The listing builds one solid part. Answer for the finished solid, in the listing's coordinates (mm). A direction names the side the tool comes from. Coordinates: 2 decimals unless noted, no trailing zeros. Loops run counter-clockwise (first coordinate to the right, second up) from the corner with the lowest first, then second, coordinate; pieces in that order, holes last. Notation, with made-up numbers: (-6, -3.5) - (41, -3.5) arc R17 ccw to (41, 3.5) - close; hole circle Ø8 at (5.25, 74). An arc over 180 degrees is marked (long way). Write each question's results on one line, items separated by ' | '. Start each with the question number.
(1) Consider line 1 (Z direction, x = 90, y = 10.5); line 2 (Y direction, x = 75, z = -9.5) (3 decimals); line 3 (X direction, y = 13.75, z = -15.5). Determine where each line is inside the solid, lowest interval first. Write a range as from..to.
(2) For faces 1 (the flat face through (0, 6, -15)), 2 (the flat face through (49, 0, -15)), 3 (the cylindrical face through (66, 12.54, -23.57)), 4 (the flat face through (14, 10, -15)), 5 (the cylindrical face through (72.5, 12.54, -15.16)), determine the directions among +Z, -Z, +X, -X, +Y, -Y from which every point of the face is accessible in a straight line to the end or side of a thin tool.
(3) Find section A-A on y = 12.75. Determine the outline of the cut face in (x, z).
(4) Find section C-C on x = 16. Determine the outline of the cut face in (y, z), then the cut area to 3 significant figures.
(5) Given pin 1 Ø2.5 at (y, z) = (12.5, -13.5) entering from +X, flat-ended and moving along its own axis, determine where the tip first touches the part or whether it passes through.
(6) Determine the mould class of faces 6 (the flat face through (50, 10, -15)), 7 (the flat face through (10, 13, -22.5)), 8 (the flat face through (100, 6, -15)) for opening direction X: released by +X, released by -X, zero draft, split by the parting line, or undercut.
(7) Find section B-B on z = -15. Determine the outline of the cut face in (x, y) (3 decimals).
(8) Find section D-D on x = 39. Determine the outline of the cut face in (y, z).
from build123d import *

# Parameters (mm, degrees)
SKETCH1_W           = 100
SKETCH1_H           = 30
BOSS_EXTRUDE1_DEPTH = 15
CUT_EXTRUDE1_DEPTH  = 5
SKETCH3_R           = 0.625
CUT_EXTRUDE2_DEPTH  = 30
CUT_EXTRUDE3_DEPTH  = 5


with BuildPart() as part:
    # Sketch1 → Boss-Extrude1 (new body)
    with BuildSketch(Plane(origin=(0, 0, 0), x_dir=(1, 0, 0), z_dir=(0, 1, 0))):
        with Locations((50, 15)):
            Rectangle(SKETCH1_W, SKETCH1_H)
    extrude(amount=BOSS_EXTRUDE1_DEPTH)

    # Sketch2 → Cut-Extrude1 (cut)
    with BuildSketch(Plane(origin=(0, 15, 0), x_dir=(1, 0, 0), z_dir=(0, 1, 0))):
        with BuildLine():
            Line((-20, 22.5), (20, 22.5))
            ThreePointArc((20, 22.5), (27.5, 15), (20, 7.5))
            Line((20, 7.5), (-20, 7.5))
            ThreePointArc((-20, 7.5), (-27.5, 15), (-20, 22.5))
        make_face()
        with BuildLine():
            Line((120, 22.5), (80, 22.5))
            ThreePointArc((80, 22.5), (72.5, 15), (80, 7.5))
            Line((80, 7.5), (120, 7.5))
            ThreePointArc((120, 7.5), (127.5, 15), (120, 22.5))
        make_face()
    extrude(amount=-CUT_EXTRUDE1_DEPTH, mode=Mode.SUBTRACT)

    # Sketch3 → Cut-Extrude2 (cut)
    with BuildSketch(Plane.XY):
        with Locations((25, 7.5)):
            Circle(SKETCH3_R)
        with Locations((75, 7.5)):
            Circle(SKETCH3_R)
    extrude(amount=-CUT_EXTRUDE2_DEPTH, mode=Mode.SUBTRACT)

    # Sketch4 → Cut-Extrude3 (cut)
    with BuildSketch(Plane(origin=(0, 15, 0), x_dir=(1, 0, 0), z_dir=(0, 1, 0))):
        with BuildLine():
            Line((37.5, 25), (62.5, 25))
            ThreePointArc((62.5, 25), (66.035533906, 23.535533906), (67.5, 20))
            Line((67.5, 20), (67.5, 10))
            ThreePointArc((67.5, 10), (66.035533906, 6.464466094), (62.5, 5))
            Line((62.5, 5), (37.5, 5))
            ThreePointArc((37.5, 5), (33.964466094, 6.464466094), (32.5, 10))
            Line((32.5, 10), (32.5, 20))
            ThreePointArc((32.5, 20), (33.964466094, 23.535533906), (37.5, 25))
        make_face()
    extrude(amount=-CUT_EXTRUDE3_DEPTH, mode=Mode.SUBTRACT)


solid = part.part
Values:
1) line 1: z = -30..-22.5, -7.5..0 | line 2: y = 0..6.875, 8.125..10 | line 3: x = 27.48..32.5, 67.5..72.52
2) face 1: +Z, -Z, -X, +Y, -Y | face 2: +Z, -Z, +X, -X, -Y | face 3: +Y | face 4: -X, +Y | face 5: +X, +Y
3) outline: (0, -30) - (100, -30) - (100, -22.5) - (80, -22.5) arc R7.5 cw to (80, -7.5) - (100, -7.5) - (100, 0) - (0, 0) - (0, -7.5) - (20, -7.5) arc R7.5 cw to (20, -22.5) - (0, -22.5) - close; hole (32.5, -20) arc R5 ccw to (37.5, -25) - (62.5, -25) arc R5 ccw to (67.5, -20) - (67.5, -10) arc R5 ccw to (62.5, -5) - (37.5, -5) arc R5 ccw to (32.5, -10) - close
4) outline: (0, -30) - (15, -30) - (15, -22.5) - (10, -22.5) - (10, -7.5) - (15, -7.5) - (15, 0) - (0, 0) - close | area: 375 mm²
5) pin 1: stops at x = 73.02
6) face 6: undercut | face 7: zero draft | face 8: released by +X
7) outline: (0, 0) - (100, 0) - (100, 10) - (72.5, 10) - (72.5, 15) - (67.5, 15) - (67.5, 10) - (32.5, 10) - (32.5, 15) - (27.5, 15) - (27.5, 10) - (0, 10) - close; hole circle Ø1.25 at (25, 7.5); hole circle Ø1.25 at (75, 7.5)
8) outline: (0, -30) - (15, -30) - (15, -25) - (10, -25) - (10, -5) - (15, -5) - (15, 0) - (0, 0) - close
